Model file for the job. Use its own axes, mm. Face numbers are marked on the shaded views. A direction names the side the tool comes from. Give positions to 0.01 mm unless a question says otherwise; leave off trailing zeros. Write each loop counter-clockwise with the first axis right and the second up, starting at its lowest first coordinate (ties: lowest second). Pieces come first, ordered by that corner, then holes. Notation, with made-up numbers: (74.5, -15) - (102.5, -15) arc R25 cw to (102.5, 6) - close; hole circle Ø11 at (15, 78.5). An arc over 180 degrees is marked (long way). Use CSV: the item, a comma, the result in double quotes.
Autodesk Inventor part; units mm, degrees
ref_plane "Plano de trabajo1" through (-239.9917, -210, 0) normal (0, -1, 0) x (1, 0, 0)
ref_plane "YZ Plane" through (0, 0, 0) normal (1, 0, 0) x (0, 1, 0)
ref_plane "XZ Plane" through (0, 0, 0) normal (0, 1, 0) x (-1, 0, 0)
sketch "Boceto1" plane through (0, 0, 0) normal (0, 0, 1) x (1, 0, 0)
  circle A0 centre (0, 0) radius 264 construction
  line L0 (-239.9917, 110) -> (239.9917, 110)
  line L1 (239.9917, 110) -> (239.9917, -110)
  line L2 (239.9917, -110) -> (-239.9917, -110)
  line L3 (-239.9917, -110) -> (-239.9917, 110)
  line L4 (-239.9917, 110) -> (239.9917, -110) construction
  line L5 (239.9917, 110) -> (-239.9917, -110) construction
  dimension "d0" = 528
  dimension "d1" = 220
extrude "Extrusión1" add sketch "Boceto1" along normal blind 30
sketch "Boceto2" plane through (0, 0, 30) normal (0, 0, 1) x (1, 0, 0)
  circle A0 centre (-189.9917, 60) radius 7.5
  line L0 (239.9917, 110) -> (-239.9917, 110) construction
  line L1 (-239.9917, 110) -> (-239.9917, -110) construction
  point P0 (0, 0)
  dimension "d4" = 15
  dimension "d5" = 50
  dimension "d6" = 50
extrude "Extrusión2" add sketch "Boceto2" along normal blind 60
mirror "Simetría1" about plane through (0, 0, 0) normal (1, 0, 0) of "Extrusión2"
mirror "Simetría2" about plane through (0, 0, 0) normal (0, 1, 0) of "Extrusión2", "Simetría1"
sketch "Boceto3" plane through (0, 0, 30) normal (0, 0, 1) x (1, 0, 0)
  circle A0 centre (0, 0) radius 80
  dimension "d17" = 160
extrude "Extrusión3" cut sketch "Boceto3" along normal through all both and the other way through all
sketch "Boceto9" plane through (-239.9917, -110, 0) normal (0, -1, 0) x (1, 0, 0)
  line L0 (0, 30) -> (479.9833, 30)
  line L1 (479.9833, 0) -> (0, 0)
  line L2 (0, 30) -> (479.9833, 30)
  line L3 (479.9833, 30) -> (479.9833, 0)
  line L4 (479.9833, 0) -> (0, 0)
  line L5 (0, 0) -> (0, 30)
  point P0 (239.9917, 0)
ref_plane "Plano de trabajo1" through (-239.9917, -210, 0) normal (0, -1, 0) x (1, 0, 0)
sketch "Boceto10" plane through (-239.9917, -210, 0) normal (0, -1, 0) x (1, 0, 0)
  line L0 (0, 0) -> (479.9833, 0) construction
  line L1 (479.9833, 0) -> (479.9833, 30) construction
  line L2 (0, 30) -> (479.9833, 30) construction
  line L3 (0, 0) -> (0, 30) construction
  line L4 (164.9917, 30) -> (314.9917, 30)
  line L5 (314.9917, 30) -> (314.9917, 0)
  line L6 (314.9917, 0) -> (164.9917, 0)
  line L7 (164.9917, 0) -> (164.9917, 30)
  point P0 (239.9917, 0)
  point P1 (239.9917, 30)
  dimension "d41" = 150
  dimension "d42" = 30
loft "Solevación1" add profiles "Boceto10" section 1 edges at (0, -110, 0) (239.9917, -110, 15) (0, -110, 30) (-239.9917, -110, 15)
sketch "Boceto11" plane through (0, 0, 0) normal (0, 0, -1) x (-1, 0, 0)
  line L0 (75, -210) -> (-75, -210)
  line L1 (-75, -210) -> (-75, -170)
  line L2 (-75, -170) -> (75, -170)
  line L3 (75, -170) -> (75, -210)
  line L4 (-75, -210) -> (75, -210)
  point P0 (0, 0)
  point P1 (0, -210)
  dimension "d48" = 150
  dimension "d49" = 40
extrude "Extrusión8" add sketch "Boceto11" along normal blind 100
sketch "Boceto12" plane through (-75, -210, 30) normal (0, -1, 0) x (1, 0, 0)
  line L0 (150, -130) -> (0, -130) construction
  line L1 (0, -30) -> (0, 0) construction
  line L2 (150, -130) -> (0, -130) construction
  line L3 (0, -130) -> (0, -30) construction
  line L4 (0, -30) -> (150, -30) construction
  line L5 (150, -30) -> (150, -130) construction
  line L6 (150, 0) -> (150, -30) construction
  line L7 (150, -30) -> (0, -130) construction
  line L8 (0, -30) -> (150, -130) construction
  circle A0 centre (75, -80) radius 31.5
  point P0 (75, -30)
  dimension "d52" = 63
extrude "Extrusión9" add sketch "Boceto12" along normal blind 20
sketch "Boceto13" plane through (0, -230, -50) normal (0, -1, 0) x (1, 0, 0)
  circle A0 centre (0, 0) radius 25 construction
  circle A1 centre (0, 25) radius 3
  circle A2 centre (0, -25) radius 3
  circle A3 centre (23.7764, -7.7254) radius 3
  circle A4 centre (14.6946, 20.2254) radius 3
  circle A5 centre (-14.6946, 20.2254) radius 3
  circle A6 centre (-23.7764, -7.7254) radius 3
  point P0 (0, 50)
  dimension "d55" = 50
  dimension "d56" = 6
  dimension "d57" = 6
  dimension "d60" = 360
extrude "Extrusión10" cut sketch "Boceto13" against normal up to next
equation "\"d0\" = 0.8 * diametro_llanta"
equation "\"d1\" = 0.333333 * diametro_llanta"
equation "\"d2\" = espesor_soporte"
equation "\"d4\" = 0.5 * espesor_soporte"
equation "\"d7\" = 2 * espesor_soporte"
equation "\"d42\" = espesor_soporte"
equation "\"ancho_llanta\" = 271000"
equation "\"espesor_soporte\" = 30"
properties part number "soporte" material "Acerito"
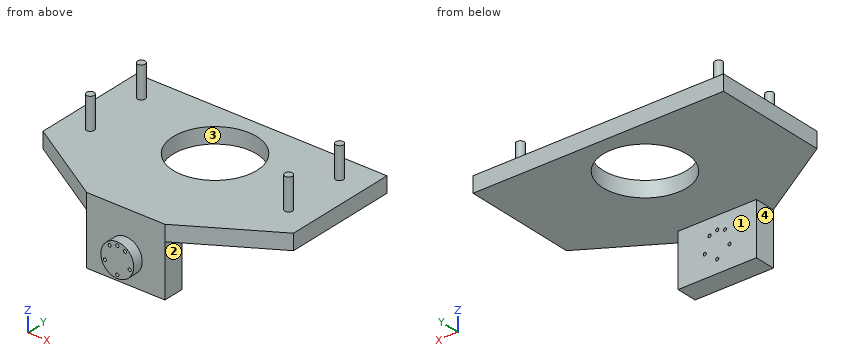
(1) Flat gauge pins, fed straight in: P1, Ø2, axis at x = -73, y = 51.5, coming from the +Z side; P2, Ø9.5, axis at x = 14.69, z = -29.77, coming from the +Y side; P3, Ø20, axis at y = -184, z = -72.5, coming from the -X side. Where does each tip first touch, or does it go through?
Checked values:
P1,"stops at z = 30"
P2,"stops at y = -170"
P3,"stops at x = -75"
(2) Saw through at A-A, the plane y = 0. List the corners of the cut face in (x, z).
Checked values:
outline,"(-239.99, 0) - (-80, 0) - (-80, 30) - (-239.99, 30) - close; (80, 0) - (239.99, 0) - (239.99, 30) - (80, 30) - close"
(3) Saw through at D-D, the plane x = 176. List the corners of the cut face in (y, z), then the cut area to 3 significant figures.
Checked values:
outline,"(-148.78, 0) - (110, 0) - (110, 30) - (-148.78, 30) - close"
area,"7,760 mm^2"
(4) Saw through at B-B, the plane z = 73. List the corners of the cut face in (x, y), then the cut area to 3 significant figures.
Checked values:
outline,"circle Ø15 at (-189.99, -60); circle Ø15 at (-189.99, 60); circle Ø15 at (189.99, -60); circle Ø15 at (189.99, 60)"
area,"707 mm^2"
(5) 3-axis set-ups, long thin cutter, end or side, ignore diameter. For the marked faces 1, 2, 3 and 4: which of +Z, -Z, +X, -X, +Y, -Y reach the whole face in a straight line?
Checked values:
face 1,"-Z, +X, -X, +Y"
face 2,"-Z, +X, +Y, -Y"
face 3,"+Z, -Z"
face 4,"-Z, -X, +Y, -Y"
(6) Saw through at C-C, the plane y = -42. List the corners of the cut face in (x, z).
Checked values:
outline,"(-239.99, 0) - (-68.09, 0) - (-68.09, 30) - (-239.99, 30) - close; (68.09, 0) - (239.99, 0) - (239.99, 30) - (68.09, 30) - close"
(7) Wall check: probe 1 along Z at (x, y) = (0, -194); probe 2 along Y at (x, z) = (0, 6); probe 3 along Z at (x, y) = (-149, 45). Give the ranges that are in metal, low to high. Write a range as [from, to].
Checked values:
probe 1,"z = [-100, -78], [-72, -28], [-22, 30]"
probe 2,"y = [-210, -80], [80, 110]"
probe 3,"z = [0, 30]"
